Model file for the job. Use its own axes, mm. Face numbers are marked on the shaded views. A direction names the side the tool comes from. Give positions to 0.01 mm unless a question says otherwise; leave off trailing zeros. Loops run counter-clockwise (first coordinate to the right, second up) from the corner with the lowest first, then second, coordinate; pieces in that order, holes last. Notation, with made-up numbers: M 30.5,-10 L 34.5,-10 A23 cw 34.5,18 Z; hole C 38,44 d7. An arc over 180 degrees is marked long. Use CSV: the item, a comma, the result in double quotes. Start each with the question number.
(1) Slice it at B-B on x = 0. List the corners of the cut face in (y, z).
(2) Slice it at D-D on y = 7.25. List the corners of the cut face in (x, z).
(3) Slice it at A-A on z = 0. List the corners of the cut face in (x, y), and give its area (3 significant figures).
(4) Wall check: line 1 along X through (y, z) = (11.5, 0); line 2 along Z through (x, y) = (0, 3). Give the ranges that are in metal, low to high. Write a range as from..to.
(5) Slice it at C-C on y = 5. List the corners of the cut face in (x, z).
(6) Tool access for the marked faces 1 and 2: list every direction of +Z, -Z, +X, -X, +Y, -Y with a clear straight run to the whole face (end or side of a thin tool).
(7) Flat gauge pins, fed straight in: P1, Ø6, axis at x = -4.5, y = 6.5, coming from the -Z side; P2, Ø3, axis at x = 0, z = 1, coming from the -Y side; P3, Ø4, axis at x = 4.5, y = 3, coming from the -Z side. Where does each tip first touch, or does it go through?
(8) Two-plate mould, pull along X, no slides. Class the marked faces 3, 4 and 5: pulls with the +X half, pulls with the -X half, needs draft (parallel to the pull), parting line crosses it, or undercut.
```python
from build123d import *

# Parameters (mm, degrees)
SKETCH1_R           = 6
BOSS_EXTRUDE1_DEPTH = 15
SKETCH2_R           = 3
CUT_EXTRUDE1_DEPTH  = 7
SKETCH3_R           = 4
CUT_EXTRUDE2_DEPTH  = 7


with BuildPart() as part:
    # Sketch1 → Boss-Extrude1 (new body)
    with BuildSketch(Plane(origin=(0, 0, 0), x_dir=(1, 0, 0), z_dir=(0, 1, 0))):
        Circle(SKETCH1_R)
    extrude(amount=BOSS_EXTRUDE1_DEPTH)

    # Sketch2 → Cut-Extrude1 (cut)
    with BuildSketch(Plane.XZ):
        Circle(SKETCH2_R)
    extrude(amount=-CUT_EXTRUDE1_DEPTH, mode=Mode.SUBTRACT)

    # Sketch3 → Cut-Extrude2 (cut)
    with BuildSketch(Plane(origin=(0, 15, 0), x_dir=(1, 0, 0), z_dir=(0, 1, 0))):
        Circle(SKETCH3_R)
    extrude(amount=-CUT_EXTRUDE2_DEPTH, mode=Mode.SUBTRACT)


solid = part.part
```
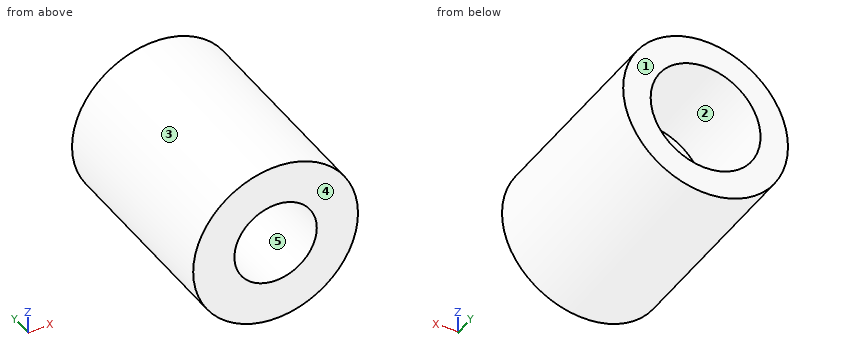
Reply:
1,outline,"M 0,-6 L 15,-6 L 15,-4 L 8,-4 L 8,4 L 15,4 L 15,6 L 0,6 L 0,3 L 7,3 L 7,-3 L 0,-3 Z"
2,outline,"C 0,0 d12"
3,outline,"M -6,0 L -3,0 L -3,7 L 3,7 L 3,0 L 6,0 L 6,15 L 4,15 L 4,8 L -4,8 L -4,15 L -6,15 Z"
3,area,"82.0 mm^2"
4,line 1,"x = -6..-4, 4..6"
4,line 2,"z = -6..-3, 3..6"
5,outline,"C 0,0 d12; hole C 0,0 d6"
6,face 1,"+Z, -Z, +X, -X, +Y"
6,face 2,"+Y"
7,P1,"stops at z = -5.81"
7,P2,"stops at y = 7"
7,P3,"stops at z = -5.45"
8,face 3,"parting line crosses it"
8,face 4,"needs draft"
8,face 5,"undercut"
